```python
from build123d import *

# Parameters (mm, degrees)
F0_R     = 5.1
F0_R_2   = 3.35
F1_DEPTH = 15
F2_START = 1.45
F0_R_3   = 11
F0_R_4   = 1.7
F2_DEPTH = 3.65


with BuildPart() as f1:
    # F0 (on Top) → F1 (new body)
    with BuildSketch(Plane.XY):
        Circle(F0_R)
        Circle(F0_R_2, mode=Mode.SUBTRACT)
    extrude(amount=F1_DEPTH)

    # F0 (on Top) → F2 (join)
    with BuildSketch(Plane.XY.offset(F2_START)):
        Circle(F0_R_3)
        with Locations((0, -8.05)):
            Circle(F0_R_4, mode=Mode.SUBTRACT)
        with Locations((-8.05, 0)):
            Circle(F0_R_4, mode=Mode.SUBTRACT)
        Circle(F0_R, mode=Mode.SUBTRACT)
        with Locations((8.05, 0)):
            Circle(F0_R_4, mode=Mode.SUBTRACT)
        with Locations((0, 8.05)):
            Circle(F0_R_4, mode=Mode.SUBTRACT)
    extrude(amount=F2_DEPTH)


solid = f1.part
```
Input: part model. Units: mm. Frame: model coordinates. A direction names the side the tool comes from. Give positions to 0.01 mm unless a question says otherwise; leave off trailing zeros. Order: outer loops, then holes, each group sorted by start corner. A loop starts at its lowest first (then second) coordinate and runs counter-clockwise, first axis right, second up. Notation, with made-up numbers: (49, -35) -> (84, -35) arc R24 ccw to (84, -23) -> close; hole circle Ø7 at (30.5, -7). An arc over 180 degrees is marked (long way). Write each question's results on one line, items separated by ' | '. Start each with the question number.
Item 1: Line query: line 1 (Y direction, x = 0, z = 2.2); line 2 (Y direction, x = 0, z = 11.5); line 3 (Z direction, x = -9.75, y = 1.5). Output: solid intervals per line, ascending.
Item 2: Cut plane C-C on x = -8.75. Return the cut outline in (y, z), then the cut area to 3 significant figures.
Item 3: Mould query, pull axis X, two halves, no side actions, for faces 1 (the cylindrical face through (2.4, -4.5, 10)), 2 (the cylindrical face through (-3.347, 0.147, 7.395)), 3 (the flat face through (2, -5, 1.45)). Classes: pulls with the +X half, pulls with the -X half, needs draft (parallel to the pull), parting line crosses it, or undercut.
Item 4: Cut plane A-A on y = 0. Return the cut outline in (x, z).
Item 5: Cut plane D-D on y = 8.05. Return the cut outline in (x, z).
Item 6: Cut plane B-B on x = -0.75. Return the cut outline in (y, z).
Item 7: Contact query for flat-ended pins moving along their axis: P1, Ø4.5, axis at x = -8.05, y = 0, coming from the -Z side; P2, Ø4.5, axis at x = 0, y = -8.05, coming from the +Z side; P3, Ø8, axis at x = -8, z = 6, coming from the -Y side. Output: stop coordinate, or through.
Item 8: Set-up query: faces 4 (the flat face through (2, -5, 5.1)), 5 (the cylindrical face through (-2.38, -10.74, 3.25)), 6 (the cylindrical face through (2.4, -4.5, 0.7)). Return all of +Z, -Z, +X, -X, +Y, -Y with unobstructed straight access to the full face (end or side cutting, diameter ignored); none if empty.
Established:
1) line 1: -11 to -9.75, -6.35 to -3.35, 3.35 to 6.35, 9.75 to 11 | line 2: -5.1 to -3.35, 3.35 to 5.1 | line 3: 1.45 to 5.1
2) outline: (-6.67, 1.45) -> (-1.55, 1.45) -> (-1.55, 5.1) -> (-6.67, 5.1) -> close; (1.55, 1.45) -> (6.67, 1.45) -> (6.67, 5.1) -> (1.55, 5.1) -> close | area: 37.4 mm^2
3) face 1: parting line crosses it | face 2: undercut | face 3: needs draft
4) outline: (-11, 1.45) -> (-9.75, 1.45) -> (-9.75, 5.1) -> (-11, 5.1) -> close; (-6.35, 1.45) -> (-5.1, 1.45) -> (-5.1, 0) -> (-3.35, 0) -> (-3.35, 15) -> (-5.1, 15) -> (-5.1, 5.1) -> (-6.35, 5.1) -> close; (3.35, 0) -> (5.1, 0) -> (5.1, 1.45) -> (6.35, 1.45) -> (6.35, 5.1) -> (5.1, 5.1) -> (5.1, 15) -> (3.35, 15) -> close; (9.75, 1.45) -> (11, 1.45) -> (11, 5.1) -> (9.75, 5.1) -> close
5) outline: (-7.5, 1.45) -> (-1.7, 1.45) -> (-1.7, 5.1) -> (-7.5, 5.1) -> close; (1.7, 1.45) -> (7.5, 1.45) -> (7.5, 5.1) -> (1.7, 5.1) -> close
6) outline: (-10.97, 1.45) -> (-9.58, 1.45) -> (-9.58, 5.1) -> (-10.97, 5.1) -> close; (-6.52, 1.45) -> (-5.04, 1.45) -> (-5.04, 0) -> (-3.26, 0) -> (-3.26, 15) -> (-5.04, 15) -> (-5.04, 5.1) -> (-6.52, 5.1) -> close; (3.26, 0) -> (5.04, 0) -> (5.04, 1.45) -> (6.52, 1.45) -> (6.52, 5.1) -> (5.04, 5.1) -> (5.04, 15) -> (3.26, 15) -> close; (9.58, 1.45) -> (10.97, 1.45) -> (10.97, 5.1) -> (9.58, 5.1) -> close
7) P1: z = 1.45 | P2: z = 5.1 | P3: y = -10.21
8) face 4: +Z | face 5: +Z, -Z | face 6: -Z
